Job drawing, mm, ordinate dimensions from the low corner. One solid piece. Coordinates: 2 decimals unless noted, no trailing zeros. One line per question, with ' | ' between items. Start each with the question number.
Item 1: Pin check, flat tip, straight feed: pin 1 (6 mm diameter, centred on x = 139, z = 127.5, fed in from -Y). Stop position of the tip, or through.
Item 2: Probe probe 1 along Z at (x, y) = (494, 2.9); probe 2 along X at (y, z) = (1.5, 6). List the from-to ranges inside material, lowest first. Write a range as [from, to].
Item 3: Two-plate mould, pull along Y, no slides. Class the marked faces 1 and 2: pulls with the +Y half, pulls with the -Y half, needs draft (parallel to the pull), parting line crosses it, or undercut.
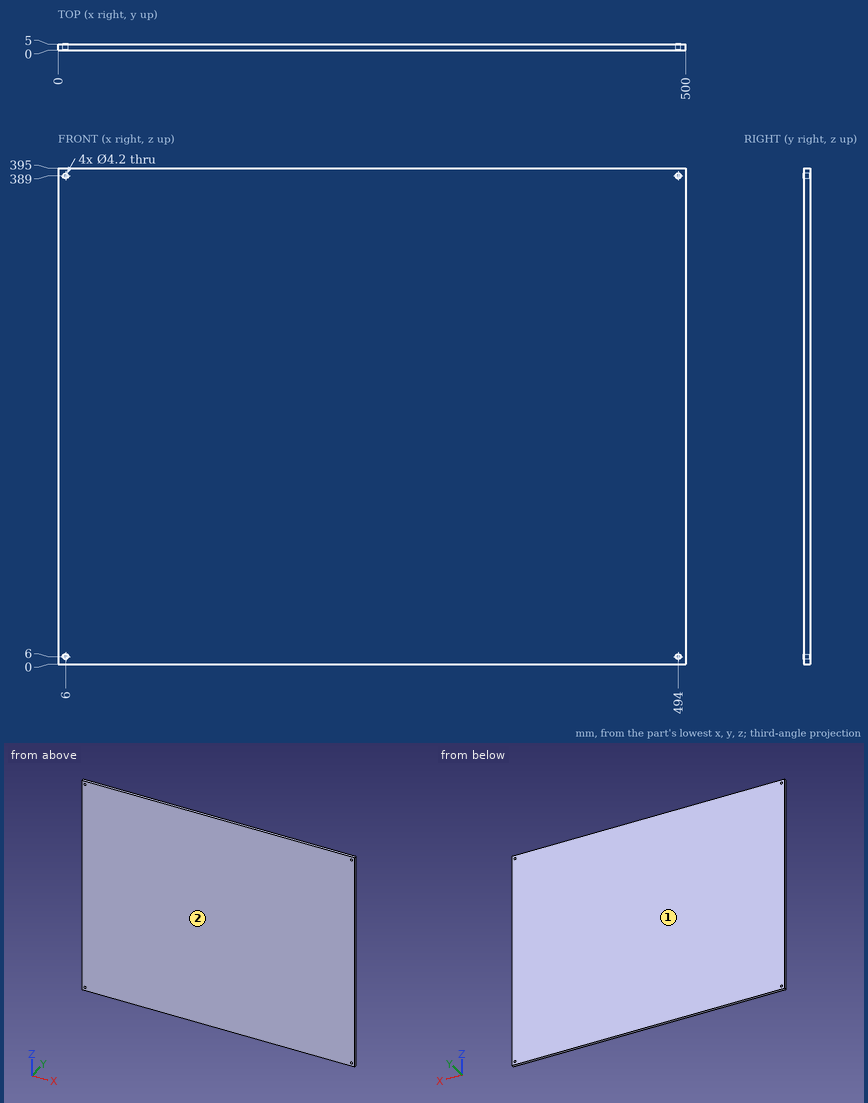
From the geometry:
1) pin 1: y = 0
2) probe 1: [0, 3.9], [8.1, 386.9], [391.1, 395] | probe 2: [0, 3.9], [8.1, 491.9], [496.1, 500]
3) face 1: pulls with the +Y half | face 2: pulls with the -Y half
